Input: part model. Units: mm. Frame: model coordinates. A direction names the side the tool comes from. Coordinates: 2 decimals unless noted, no trailing zeros. Loops run counter-clockwise (first coordinate to the right, second up) from the corner with the lowest first, then second, coordinate; pieces in that order, holes last.
(1) Mould query, pull axis X, two halves, no side actions, for faces 1 (the face through (9.28, 32.84, 2.96)), 2 (the face through (-67.328, 12, 3)), 3 (the face through (83.672, 12, 3)). Classes: released by +X, released by -X, zero draft, split by the parting line, or undercut.
(2) Section A-A, the plane x = -41.5. Return loops of the section in (y, z), then the cut area to 4 significant figures.
(3) Section C-C, the plane y = 51. Return loops of the section in (x, z), then the cut area to 3 significant figures.
(4) Contact query for flat-ended pins moving along their axis: P1, Ø2, axis at x = -53, z = 1.5, coming from the +Y side; P2, Ø10, axis at x = 64.5, y = 34.5, coming from the -Z side; P3, Ø0.6, axis at y = -4, z = 1.5, coming from the -X side. Output: stop coordinate, or through.
(5) Line query: L1, parallel to Y at x = 72, z = 3.9; L2, parallel to Y at x = -57.5, z = 4.6; L3, parallel to X at y = 62.5, z = 4.05. Output: solid intervals per line, ascending.
(6) Section B-B, the plane z = 1.1. Give the number of separate pieces and of enclosed holes in the cut face, then the cut area to 3 significant figures.
(7) Set-up query: faces 4 (the face through (23, 71.187, 3)), 5 (the face through (63, 71.187, 3)), 6 (the face through (-61.328, -6, 3)), 7 (the face through (77.672, -96, 3)). Return all of +Z, -Z, +X, -X, +Y, -Y with unobstructed straight access to the full face (end or side cutting, diameter ignored); none if empty.
Autodesk Inventor part; units mm, degrees
ref_plane "YZ Plane" through (0, 0, 0) normal (1, 0, 0) x (0, 1, 0)
ref_plane "XZ Plane" through (0, 0, 0) normal (0, 1, 0) x (-1, 0, 0)
ref_plane "XY Plane" through (0, 0, 0) normal (0, 0, 1) x (1, 0, 0)
sketch "Sketch1" plane through (0, 0, 0) normal (0, 0, 1) x (1, 0, 0)
  circle A0 centre (8.172, 30.7121) radius 2.4
  circle A1 centre (67.672, -114.2879) radius 2.4
  circle A2 centre (-51.328, -114.2879) radius 2.4
  line L0 (-61.328, 71.2121) -> (-61.328, 18.0121)
  line L1 (-61.328, 18.0121) -> (-67.328, 17.9121)
  line L2 (-67.328, 17.9121) -> (-67.328, 6.1121)
  line L3 (-67.328, 6.1121) -> (-61.328, 6.0121)
  line L4 (-61.328, 6.0121) -> (-61.328, -0.2879)
  line L5 (-61.328, -0.2879) -> (-54.328, -0.2879)
  line L6 (-54.328, -0.2879) -> (-54.328, 0.9621)
  line L7 (-54.328, 0.9621) -> (-52.528, 0.9621)
  line L8 (-52.528, 0.9621) -> (-52.528, -0.2879)
  line L9 (-52.528, -0.2879) -> (-49.528, -0.2879)
  line L10 (-49.528, -0.2879) -> (-49.528, -3.2879)
  line L11 (-49.528, -3.2879) -> (-52.528, -3.2879)
  line L12 (-52.528, -3.2879) -> (-52.528, -4.5379)
  line L13 (-52.528, -4.5379) -> (-54.328, -4.5379)
  line L14 (-54.328, -4.5379) -> (-54.328, -3.2879)
  line L15 (-54.328, -3.2879) -> (-61.328, -3.2879)
  line L16 (-61.328, -3.2879) -> (-61.328, -9.7879)
  line L17 (-61.328, -9.7879) -> (-67.328, -9.8879)
  line L18 (-67.328, -9.8879) -> (-67.328, -21.6879)
  line L19 (-67.328, -21.6879) -> (-61.328, -21.7879)
  line L20 (-61.328, -21.7879) -> (-61.328, -71.4879)
  line L21 (-61.328, -71.4879) -> (-67.328, -71.5879)
  line L22 (-67.328, -71.5879) -> (-67.328, -83.3879)
  line L23 (-67.328, -83.3879) -> (-61.328, -83.4879)
  line L24 (-61.328, -83.4879) -> (-61.328, -89.7879)
  line L25 (-61.328, -89.7879) -> (-54.328, -89.7879)
  line L26 (-54.328, -89.7879) -> (-54.328, -88.5379)
  line L27 (-54.328, -88.5379) -> (-52.528, -88.5379)
  line L28 (-52.528, -88.5379) -> (-52.528, -89.7879)
  line L29 (-52.528, -89.7879) -> (-49.528, -89.7879)
  line L30 (-49.528, -89.7879) -> (-49.528, -92.7879)
  line L31 (-49.528, -92.7879) -> (-52.528, -92.7879)
  line L32 (-52.528, -92.7879) -> (-52.528, -94.0379)
  line L33 (-52.528, -94.0379) -> (-54.328, -94.0379)
  line L34 (-54.328, -94.0379) -> (-54.328, -92.7879)
  line L35 (-54.328, -92.7879) -> (-61.328, -92.7879)
  line L36 (-61.328, -92.7879) -> (-61.328, -99.2879)
  line L37 (-61.328, -99.2879) -> (-67.328, -99.3879)
  line L38 (-67.328, -99.3879) -> (-67.328, -111.1879)
  line L39 (-67.328, -111.1879) -> (-61.328, -111.2879)
  line L40 (-61.328, -111.2879) -> (-61.328, -126.2879)
  line L41 (-61.328, -126.2879) -> (77.672, -126.2879)
  line L42 (77.672, -126.2879) -> (77.672, -111.2879)
  line L43 (77.672, -111.2879) -> (83.672, -111.1879)
  line L44 (83.672, -111.1879) -> (83.672, -99.3879)
  line L45 (83.672, -99.3879) -> (77.672, -99.2879)
  line L46 (77.672, -99.2879) -> (77.672, -92.9879)
  line L47 (77.672, -92.9879) -> (70.672, -92.9879)
  line L48 (70.672, -92.9879) -> (70.672, -94.2379)
  line L49 (70.672, -94.2379) -> (68.872, -94.2379)
  line L50 (68.872, -94.2379) -> (68.872, -92.9879)
  line L51 (68.872, -92.9879) -> (65.872, -92.9879)
  line L52 (65.872, -92.9879) -> (65.872, -89.9879)
  line L53 (65.872, -89.9879) -> (68.872, -89.9879)
  line L54 (68.872, -89.9879) -> (68.872, -88.7379)
  line L55 (68.872, -88.7379) -> (70.672, -88.7379)
  line L56 (70.672, -88.7379) -> (70.672, -89.9879)
  line L57 (70.672, -89.9879) -> (77.672, -89.9879)
  line L58 (77.672, -89.9879) -> (77.672, -83.4879)
  line L59 (77.672, -83.4879) -> (83.672, -83.3879)
  line L60 (83.672, -83.3879) -> (83.672, -71.5879)
  line L61 (83.672, -71.5879) -> (77.672, -71.4879)
  line L62 (77.672, -71.4879) -> (77.672, -21.6879)
  line L63 (77.672, -21.6879) -> (83.672, -21.5879)
  line L64 (83.672, -21.5879) -> (83.672, -9.7879)
  line L65 (83.672, -9.7879) -> (77.672, -9.6879)
  line L66 (77.672, -9.6879) -> (77.672, -3.3879)
  line L67 (77.672, -3.3879) -> (70.672, -3.3879)
  line L68 (70.672, -3.3879) -> (70.672, -4.6379)
  line L69 (70.672, -4.6379) -> (68.872, -4.6379)
  line L70 (68.872, -4.6379) -> (68.872, -3.3879)
  line L71 (68.872, -3.3879) -> (65.872, -3.3879)
  line L72 (65.872, -3.3879) -> (65.872, -0.3879)
  line L73 (65.872, -0.3879) -> (68.872, -0.3879)
  line L74 (68.872, -0.3879) -> (68.872, 0.8621)
  line L75 (68.872, 0.8621) -> (70.672, 0.8621)
  line L76 (70.672, 0.8621) -> (70.672, -0.3879)
  line L77 (70.672, -0.3879) -> (77.672, -0.3879)
  line L78 (77.672, -0.3879) -> (77.672, 6.1121)
  line L79 (77.672, 6.1121) -> (83.672, 6.2121)
  line L80 (83.672, 6.2121) -> (83.672, 18.0121)
  line L81 (83.672, 18.0121) -> (77.672, 18.0868)
  line L82 (77.672, 18.0868) -> (77.672, 71.1868)
  line L83 (77.672, 71.1868) -> (47.672, 71.1868)
  line L84 (47.672, 71.1868) -> (47.572, 77.1868)
  line L85 (47.572, 77.1868) -> (35.772, 77.1868)
  line L86 (35.772, 77.1868) -> (35.672, 71.1868)
  line L87 (35.672, 71.1868) -> (9.672, 71.1868)
  line L88 (9.672, 71.1868) -> (9.672, 64.1868)
  line L89 (9.672, 64.1868) -> (10.922, 64.1868)
  line L90 (10.922, 64.1868) -> (10.922, 62.3868)
  line L91 (10.922, 62.3868) -> (9.672, 62.3868)
  line L92 (9.672, 62.3868) -> (9.672, 60.9868)
  line L93 (9.672, 60.9868) -> (6.672, 60.9868)
  line L94 (6.672, 60.9868) -> (6.672, 62.3868)
  line L95 (6.672, 62.3868) -> (5.422, 62.3868)
  line L96 (5.422, 62.3868) -> (5.422, 64.1868)
  line L97 (5.422, 64.1868) -> (6.672, 64.1868)
  line L98 (6.672, 64.1868) -> (6.672, 71.1868)
  line L99 (6.672, 71.1868) -> (-19.328, 71.1868)
  line L100 (-19.328, 71.1868) -> (-19.428, 77.2121)
  line L101 (-19.428, 77.2121) -> (-31.228, 77.2121)
  line L102 (-31.228, 77.2121) -> (-31.328, 71.2121)
  line L103 (-31.328, 71.2121) -> (-61.328, 71.2121)
  point P0 (0, 0)
  point P1 (0, 0)
extrude "Extrusion1" add sketch "Sketch1" along normal blind 6
properties part number "yCarPlate"
Report:
1. face 1: undercut
1. face 2: released by -X
1. face 3: released by +X
2. outline: (-126.29, 0) - (71.21, 0) - (71.21, 6) - (-126.29, 6) - close
2. area: 1,185 mm2
3. outline: (-61.33, 0) - (77.67, 0) - (77.67, 6) - (-61.33, 6) - close
3. area: 834 mm2
4. P1: stops at y = 71.21
4. P2: stops at z = 0
4. P3: stops at x = -61.33
5. L1: y = -126.29 to -92.99, -89.99 to -3.39, -0.39 to 71.19
5. L2: y = -126.29 to -92.79, -89.79 to -3.29, -0.29 to 71.21
5. L3: x = -61.33 to 5.42, 10.92 to 77.67
6. separate pieces: 1
6. enclosed holes: 3
6. area: 27,900 mm2
7. face 4: +Z, -Z, +Y
7. face 5: +Z, -Z, +X, +Y
7. face 6: +Z, -Z, -X
7. face 7: +Z, -Z, +X
